The listing builds one solid part. Answer for the finished solid, in the listing's coordinates (mm). Face numbers are marked on the shaded views. A direction names the side the tool comes from. Coordinates: 2 decimals unless noted, no trailing zeros. Order: outer loops, then holes, each group sorted by start corner. A loop starts at its lowest first (then second) coordinate and runs counter-clockwise, first axis right, second up. Notation, with made-up numbers: (38, 70) - (66, 70) arc R17 ccw to (66, 81) - close; hole circle Ø2 at (-30, 10). An arc over 180 degrees is marked (long way). Use a Markdown table: item, result. Add a question column.
Item 1: The mould has two halves that part along Z. Classify the marked faces 3, 4, 5 and 6: released by +Z, released by -Z, zero draft, split by the parting line, or undercut.
Item 2: The part is cut by section C-C, the plane x = 45. State how many separate pieces and enclosed holes the cut face has, then the cut area to 3 significant figures.
Item 3: For the marked faces 1 and 2, determine the directions among +Z, -Z, +X, -X, +Y, -Y from which every point of the face is accessible in a straight line to the end or side of a thin tool.
Item 4: Find the intervals of material crossed by line 1 along X through (y, z) = (5.75, -49); line 2 along Z through (x, y) = (-16.5, 2.5); line 3 along Z through (x, y) = (35, 11.5), in increasing order.
Item 5: The part is cut by section A-A, the plane x = 0. Give the vertices of the cut face in (y, z) (3 decimals).
Item 6: Flat-ended cylindrical pins translate along their axes: P1, Ø4, axis at y = 2, z = -12, coming from the +X side; P2, Ø6, axis at y = 3.5, z = 56.5, coming from the +X side; P3, Ø5.5, axis at x = 0, z = 0, coming from the +Y side; P4, Ø6, axis at x = 36, y = 4.5, coming from the -Z side. Find the tip coordinate at first contact, or state that the pin passes through.
Item 7: The part is cut by section B-B, the plane z = 46. Give the vertices of the cut face in (x, y).
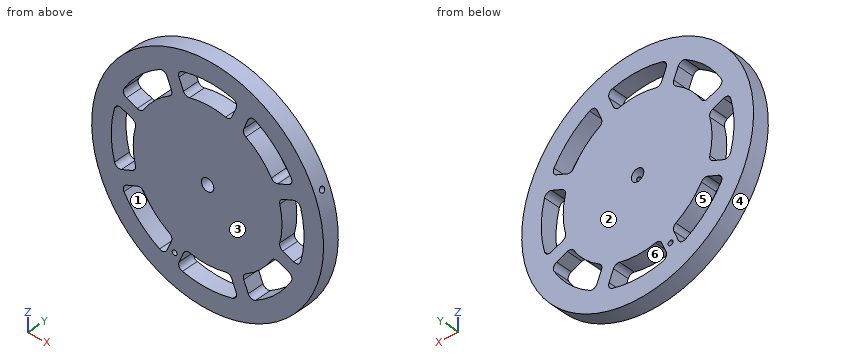
from build123d import *

# Parameters (mm, degrees)
SKETCH2_W                = 89.05
SKETCH2_H                = 12.7
F_10_24_TAPPED_HOLE2_D   = 3.7973
CUT_EXTRUDE1_DEPTH       = 13.7
FILLET1_R                = 4
CIRPATTERN4_COUNT        = 8
FILLET1_OF_CIRPATTERN4_R = 4
SKETCH15_W               = 2.0447
SKETCH15_H               = 116.349432022
SKETCH22_R               = 4.765
CUT_EXTRUDE4_DEPTH       = 12.8


with BuildPart() as part:
    # Sketch2 → Revolve1 (revolve)
    with BuildSketch(Plane(origin=(0, 0, 0), x_dir=(0, 0, -1), z_dir=(1, 0, 0))):
        with Locations((-44.525, 6.35)):
            Rectangle(SKETCH2_W, SKETCH2_H)
    revolve(axis=Axis((0, -0.888756804, 0), (0, 1, 0)))

    # #10-24 Tapped Hole2 (through all)
    with Locations(Plane(origin=(0, 12.7, 0), x_dir=(1, 0, 0), z_dir=(0, 1, 0))):
        with Locations((-25.333643223, 61.160825052)):
            Hole(F_10_24_TAPPED_HOLE2_D / 2)

    # Sketch8 → Cut-Extrude1 (cut, through all)
    with BuildSketch(Plane(origin=(0, 12.7, 0), x_dir=(1, 0, 0), z_dir=(0, 1, 0))):
        with BuildLine():
            Line((-17.167098173, 54.510670885), (-23.653637882, 70.170563023))
            ThreePointArc((-23.653637882, 70.170563023), (0, 74.05), (23.653637882, 70.170563023))
            Line((23.653637882, 70.170563023), (17.167098173, 54.510670885))
            ThreePointArc((17.167098173, 54.510670885), (0, 57.15), (-17.167098173, 54.510670885))
        make_face()
    cut_extrude1 = extrude(amount=-CUT_EXTRUDE1_DEPTH, mode=Mode.SUBTRACT)

    # Fillet1
    fillet1_edges = [part.edges().sort_by_distance(p)[0] for p in [
        (17.167098173, 6.35, -54.510670885),
        (-17.167098173, 6.35, -54.510670885),
        (-23.653637882, 6.35, -70.170563023),
        (23.653637882, 6.35, -70.170563023),
    ]]
    fillet(fillet1_edges, radius=FILLET1_R)

    # CirPattern4: Cut-Extrude1 ×8 about axis
    cirpattern4_axis = Axis((0, 0, 0), (0, 1, 0))
    for i in range(1, CIRPATTERN4_COUNT):
        add(cut_extrude1.rotate(cirpattern4_axis, i * 360 / CIRPATTERN4_COUNT), mode=Mode.SUBTRACT)

    # Fillet1 of CirPattern4
    fillet1_of_cirpattern4_edges = [part.edges().sort_by_distance(p)[0] for p in [
        (-26.405893498, 6.35, -50.683836561),
        (-50.683836561, 6.35, -26.405893498),
        (-66.343728699, 6.35, -32.892433207),
        (-32.892433207, 6.35, -66.343728699),
        (-54.510670885, 6.35, -17.167098173),
        (-54.510670885, 6.35, 17.167098173),
        (-70.170563023, 6.35, 23.653637882),
        (-70.170563023, 6.35, -23.653637882),
        (-50.683836561, 6.35, 26.405893498),
        (-26.405893498, 6.35, 50.683836561),
        (-32.892433207, 6.35, 66.343728699),
        (-66.343728699, 6.35, 32.892433207),
        (-17.167098173, 6.35, 54.510670885),
        (17.167098173, 6.35, 54.510670885),
        (23.653637882, 6.35, 70.170563023),
        (-23.653637882, 6.35, 70.170563023),
        (26.405893498, 6.35, 50.683836561),
        (50.683836561, 6.35, 26.405893498),
        (66.343728699, 6.35, 32.892433207),
        (32.892433207, 6.35, 66.343728699),
        (54.510670885, 6.35, 17.167098173),
        (54.510670885, 6.35, -17.167098173),
        (70.170563023, 6.35, -23.653637882),
        (70.170563023, 6.35, 23.653637882),
        (50.683836561, 6.35, -26.405893498),
        (26.405893498, 6.35, -50.683836561),
        (32.892433207, 6.35, -66.343728699),
        (66.343728699, 6.35, -32.892433207),
    ]]
    fillet(fillet1_of_cirpattern4_edges, radius=FILLET1_OF_CIRPATTERN4_R)

    # Sketch15 → #20 (0.161) Diameter Hole1 (revolve, cut)
    with BuildSketch(Plane(origin=(0, 6.35, 0), x_dir=(-0.382683432, 0, 0.923879533), z_dir=(0, 1, 0))):
        with Locations((1.02235, 58.174716011)):
            Rectangle(SKETCH15_W, SKETCH15_H)
    revolve(axis=Axis((-5.866635031, 6.35, -2.430039796), (0.923879533, 0, 0.382683432)), mode=Mode.SUBTRACT)

    # Sketch22 → Cut-Extrude4 (cut)
    with BuildSketch(Plane(origin=(0, 12.7, 0), x_dir=(1, 0, 0), z_dir=(0, 1, 0))):
        Circle(SKETCH22_R)
    extrude(amount=-CUT_EXTRUDE4_DEPTH, mode=Mode.SUBTRACT)


solid = part.part
Solution:
| question | item | result |
|---|---|---|
| 1 | face 3 | zero draft |
| 1 | face 4 | split by the parting line |
| 1 | face 5 | undercut |
| 1 | face 6 | undercut |
| 2 | separate pieces | 3 |
| 2 | enclosed holes | 1 |
| 2 | area | 1,340 mm2 |
| 3 | face 1 | +Y, -Y |
| 3 | face 2 | +Z, -Z, +X, -X, +Y |
| 4 | line 1 | x = -74.36 to -55.52, -29.41 to 29.41, 55.52 to 74.36 |
| 4 | line 2 | z = -87.51 to -72.19, -55.69 to 55.69, 72.19 to 87.51 |
| 4 | line 3 | z = -81.88 to -64.74, -45.18 to 45.18, 64.74 to 81.88 |
| 5 | outline | (0, -89.05) - (12.7, -89.05) - (12.7, -74.05) - (0, -74.05) - close; (0, -57.15) - (12.7, -57.15) - (12.7, -4.765) - (0, -4.765) - close; (0, 4.765) - (12.7, 4.765) - (12.7, 57.15) - (0, 57.15) - close; (0, 74.05) - (12.7, 74.05) - (12.7, 89.05) - (0, 89.05) - close |
| 6 | P1 | stops at x = 88.49 |
| 6 | P2 | stops at x = 71.19 |
| 6 | P3 | passes through |
| 6 | P4 | stops at z = -82.71 |
| 7 | outline | (-76.25, 0) - (-58.03, 0) - (-58.03, 12.7) - (-76.25, 12.7) - close; (-33.91, 0) - (33.91, 0) - (33.91, 12.7) - (-33.91, 12.7) - close; (58.03, 0) - (76.25, 0) - (76.25, 12.7) - (58.03, 12.7) - close |
